```python
from build123d import *

# Parameters (mm, degrees)
F0_W     = 165.1
F0_H     = 127
F1_DEPTH = 9.525
F2_D     = 38.1
F3_W     = 50.8
F3_H     = 50.8
F4_DEPTH = 63.5
F5_R     = 25.4


with BuildPart() as f1:
    # F0 (on Front) → F1 (new body)
    with BuildSketch(Plane.XZ):
        Rectangle(F0_W, F0_H)
    extrude(amount=F1_DEPTH)

    # F2 (through all)
    with Locations(Plane(origin=(0, 0, 0), x_dir=(1, 0, 0), z_dir=(0, 1, 0))):
        with Locations((0, 0)):
            Hole(F2_D / 2)

    # F3 (on Front) → F4 (join)
    with BuildSketch(Plane.XZ):
        with Locations((-57.190858, 38.099989)):
            Rectangle(F3_W, F3_H)
        with Locations((57.109142, 38.099989)):
            Rectangle(F3_W, F3_H)
    extrude(amount=F4_DEPTH)

    # F5
    f5_edges = [f1.edges().sort_by_distance(p)[0] for p in [
        (-31.790858, -36.5125, 12.699989),
        (31.709142, -36.5125, 12.699989),
    ]]
    fillet(f5_edges, radius=F5_R)


solid = f1.part
```
Geometry check sheet. Reference: the model listing, model coordinates, mm. A direction names the side the tool comes from. Round coordinates to 2 decimals unless told otherwise and drop trailing zeros. Loops run counter-clockwise (first coordinate to the right, second up) from the corner with the lowest first, then second, coordinate; pieces in that order, holes last. Notation, with made-up numbers: (-11.75, 73.5) - (-7.75, 73.5) arc R24 ccw to (-7.75, 95.5) - close; hole circle Ø8 at (-35.75, 82). An arc over 180 degrees is marked (long way). Write each question's results on one line, items separated by ' | '. Start each with the question number.
Q1. Cross-section at C-C on x = 0. Enter the section's corners in (y, z) (3 decimals).
Q2. Release check for a two-part mould opening along X. For faces 4 (the flat face through (-82.591, -31, 38)), 5 (the flat face through (-1, -9.525, -27)), 6 (the flat face through (-1, -5, 63.5)) record: +X half, -X half, draft (parallel to the pull), parting line (faces both ways), or undercut.
Q3. Cross-section at A-A on y = -38.5. Enter the section's corners in (x, z).
Q4. Access from +Z, -Z, +X, -X, +Y, -Y to the whole of each face (thin tool, end or side, straight path). Record for faces 1 (the flat face through (70, -36, 12.7)), 2 (the cylindrical face through (-39.43, -36.89, 19.94)), 3 (the flat face through (31.709, -36, 51)).
Q5. Gauge pin test, flat ends, axial feed: P1, Ø12.5, axis at x = 70, y = -29.5, coming from the -Z side; P2, Ø1, axis at y = -11, z = -13, coming from the -X side; P3, Ø7.5, axis at y = -4, z = -9.5, coming from the -X side; P4, Ø12.5, axis at y = -33.5, z = 56, coming from the +X side. Record the tip position at first contact, or that the pin passes through.
Q6. Cross-section at B-B on z = 0. Enter the section's corners in (x, y) (3 decimals).
Q7. Thickness scan on line 1 (X direction, y = -44.5, z = 41.5); line 2 (Z direction, x = 0, y = -3); line 3 (Y direction, x = -53.5, z = 7.5) (3 decimals). Record the ranges inside material, lowest first. Write a range as [from, to].
Answers below:
1) outline: (-9.525, -63.5) - (0, -63.5) - (0, -19.05) - (-9.525, -19.05) - close; (-9.525, 19.05) - (0, 19.05) - (0, 63.5) - (-9.525, 63.5) - close
2) face 4: -X half | face 5: undercut | face 6: draft
3) outline: (-82.59, 12.7) - (-57.19, 12.7) arc R25.4 ccw to (-31.79, 38.1) - (-31.79, 63.5) - (-82.59, 63.5) - close; (31.71, 38.1) arc R25.4 ccw to (57.11, 12.7) - (82.51, 12.7) - (82.51, 63.5) - (31.71, 63.5) - close
4) face 1: -Z, +X, -X, -Y | face 2: -Z, -Y | face 3: +Z, -Z, -Y
5) P1: stops at z = 12.7 | P2: passes through | P3: stops at x = -82.55 | P4: stops at x = 82.51
6) outline: (-82.55, -9.525) - (-19.05, -9.525) - (-19.05, 0) - (-82.55, 0) - close; (19.05, -9.525) - (82.55, -9.525) - (82.55, 0) - (19.05, 0) - close
7) line 1: x = [-82.59, -31.79], [31.71, 82.51] | line 2: z = [-63.5, -19.05], [19.05, 63.5] | line 3: y = [-9.525, 0]
